from build123d import *

# Parameters (mm, degrees)
SKETCH_1_W             = 160
SKETCH_1_H             = 45
EXTRUDE_1_DEPTH        = 52
SKETCH_2_R             = 15
CUT_EXTRUDE_1_DEPTH    = 10
PATTERN_LINEAR_2_COUNT = 3
PATTERN_LINEAR_2_PITCH = 32
PATTERN_LINEAR_3_COUNT = 3
PATTERN_LINEAR_3_PITCH = 32
FILLET_1_R             = 20
FILLET_2_R             = 10


with BuildPart() as part:
    # 스케치1 → 보스-돌출1 (new body)
    with BuildSketch(Plane.XY):
        Rectangle(SKETCH_1_W, SKETCH_1_H)
    extrude(amount=EXTRUDE_1_DEPTH)

    # 스케치2 → 컷-돌출1 (cut)
    with BuildSketch(Plane(origin=(0, 0, 0), x_dir=(-1, 0, 0), z_dir=(0, 0, -1))):
        Circle(SKETCH_2_R)
    cut_extrude_1 = extrude(amount=-CUT_EXTRUDE_1_DEPTH, mode=Mode.SUBTRACT)

    # 선형 패턴2: 컷-돌출1 ×3
    with Locations(*[(-i * PATTERN_LINEAR_2_PITCH, 0, 0) for i in range(1, PATTERN_LINEAR_2_COUNT)]):
        add(cut_extrude_1, mode=Mode.SUBTRACT)

    # 선형 패턴3: 컷-돌출1 ×3
    with Locations(*[(i * PATTERN_LINEAR_3_PITCH, 0, 0) for i in range(1, PATTERN_LINEAR_3_COUNT)]):
        add(cut_extrude_1, mode=Mode.SUBTRACT)

    # 필렛1
    fillet_1_edges = [part.edges().sort_by_distance(p)[0] for p in [
        (0, -22.5, 52),
        (0, 22.5, 52),
    ]]
    fillet(fillet_1_edges, radius=FILLET_1_R)

    # 필렛2
    fillet_2_edges = [part.edges().sort_by_distance(p)[0] for p in [
        (80, 0, 52),
        (-80, 0, 52),
        (80, 22.5, 16),
        (80, -22.5, 16),
        (80, 16.642135624, 46.142135624),
        (80, -16.642135624, 46.142135624),
        (-80, -22.5, 16),
        (-80, 22.5, 16),
        (-80, 16.642135624, 46.142135624),
        (-80, -16.642135624, 46.142135624),
    ]]
    fillet(fillet_2_edges, radius=FILLET_2_R)


solid = part.part
The listing builds one solid part. Answer for the finished solid, in the listing's coordinates (mm). A direction names the side the tool comes from. Round coordinates to 2 decimals unless told otherwise and drop trailing zeros. Loops run counter-clockwise (first coordinate to the right, second up) from the corner with the lowest first, then second, coordinate; pieces in that order, holes last. Notation, with made-up numbers: M -38.5,55 L -28.5,55 A23 cw -28.5,94 Z; hole C -15.5,66 d3. An arc over 180 degrees is marked long. Write each question's results on one line, items separated by ' | '. Start each with the question number.
1) Determine the mould class of faces 1 (the flat face through (64, 0, 10)), 2 (the cylindrical face through (-77.15, 0.04, 48.99)), 3 (the cylindrical face through (0.98, 16.797, 45.986)) for opening direction X: pulls with the +X half, pulls with the -X half, needs draft (parallel to the pull), parting line crosses it, or undercut.
2) Find section B-B on x = -32. Write down the section's boundary in (y, z).
3) Which of the six approach directions +Z, -Z, +X, -X, +Y, -Y give full straight-line access (tool end or side, diameter ignored) to faces 4 (the flat face through (-80, 0, 21)), 5 (the cylindrical face through (78.985, 0.66, 4.93))?
4) Find section A-A on z = 3. Write down the section's boundary in (x, y).
5) Straight lines are drawn through the part: probe 1 along Y at (x, z) = (-64, 4.75); probe 2 along X at (y, z) = (3.5, 9); probe 3 along Y at (x, z) = (51.5, 8). For each, find the intervals that lie inside material, in ascending order.
6) Each of these flat-tipped pins is pushed along its axis until it touches: pin 1 (9 mm diameter, centred on x = -33, y = 7.5, fed in from -Z); pin 2 (1 mm diameter, centred on y = -10.5, z = 43.5, fed in from +X); pin 3 (2 mm diameter, centred on y = -14, z = 30.5, fed in from +X). Where does it stop, or does it pass through?
7) Find section C-C on x = 4.5. Write down the section's boundary in (y, z), plus the area to 3 significant figures.
Final values:
1) face 1: undercut | face 2: pulls with the -X half | face 3: needs draft
2) outline: M -22.5,0 L -15,0 L -15,10 L 15,10 L 15,0 L 22.5,0 L 22.5,32 A20 ccw 2.5,52 L -2.5,52 A20 ccw -22.5,32 Z
3) face 4: +Z, -Z, -X, +Y, -Y | face 5: -Z
4) outline: M -80,-12.5 A10 ccw -70,-22.5 L 70,-22.5 A10 ccw 80,-12.5 L 80,12.5 A10 ccw 70,22.5 L -70,22.5 A10 ccw -80,12.5 Z; hole C -64,0 d30; hole C -32,0 d30; hole C 0,0 d30; hole C 32,0 d30; hole C 64,0 d30
5) probe 1: -22.5 to -15, 15 to 22.5 | probe 2: -80 to -78.59, -49.41 to -46.59, -17.41 to -14.59, 14.59 to 17.41, 46.59 to 49.41, 78.59 to 80 | probe 3: -22.5 to -8.29, 8.29 to 22.5
6) pin 1: z = 10 | pin 2: x = 79.36 | pin 3: x = 79.99
7) outline: M -22.5,0 L -14.31,0 L -14.31,10 L 14.31,10 L 14.31,0 L 22.5,0 L 22.5,32 A20 ccw 2.5,52 L -2.5,52 A20 ccw -22.5,32 Z | area: 1,880 mm²
